from build123d import *

# Parameters (mm, degrees)
SKETCH1_R           = 7
BOSS_EXTRUDE1_DEPTH = 20
BOSS_EXTRUDE2_START = 1
SKETCH2_R           = 7
SKETCH2_R_2         = 2.05
BOSS_EXTRUDE2_DEPTH = 1


with BuildPart() as part:
    # Sketch1 → Boss-Extrude1 (new body)
    with BuildSketch(Plane(origin=(0, 0, 0), x_dir=(1, 0, 0), z_dir=(0, 1, 0))):
        with Locations(Location((0, 0, 0), (0, 0, 270))):
            Circle(SKETCH1_R)
        Polygon((0, 6.985938257), (-6.05, 3.492969129), (-6.05, -3.492969129), (0, -6.985938257), (6.05, -3.492969129), (6.05, 3.492969129), align=None, mode=Mode.SUBTRACT)
    extrude(amount=BOSS_EXTRUDE1_DEPTH)

    # Sketch2 → Boss-Extrude2 (add)
    with BuildSketch(Plane.XZ.offset(BOSS_EXTRUDE2_START)):
        with Locations(Location((0, 0, 0), (0, 0, 270))):
            Circle(SKETCH2_R)
        with Locations(Location((0, 0, 0), (0, 0, 270))):
            Circle(SKETCH2_R_2, mode=Mode.SUBTRACT)
    extrude(amount=-BOSS_EXTRUDE2_DEPTH)


solid = part.part
Geometry check sheet. Reference: the model listing, model coordinates, mm. A direction names the side the tool comes from. Round coordinates to 2 decimals unless told otherwise and drop trailing zeros. Order: outer loops, then holes, each group sorted by start corner. A loop starts at its lowest first (then second) coordinate and runs counter-clockwise, first axis right, second up. Notation, with made-up numbers: M 76.5,46.5 L 92.5,46.5 A20 ccw 92.5,68.5 Z; hole C 26.25,-22.75 d2. An arc over 180 degrees is marked long. Answer in a Markdown table with one row per item.
(1) Draft check along X on faces 3 (the face through (-3.067, 9.86, 5.215)), 4 (the face through (2, -1, -1)). Enter one of: released by +X, released by -X, zero draft, split by the parting line, or undercut.
Responses:
| item | result |
|---|---|
| face 3 | undercut |
| face 4 | zero draft |
(2) Sectioned sample at D-D, the plane x = -5. Record the cut outline in (y, z), and give its area (3 significant figures).
Responses:
| item | result |
|---|---|
| outline | M -1,-4.9 L 20,-4.9 L 20,-4.1 L 0,-4.1 L 0,4.1 L 20,4.1 L 20,4.9 L -1,4.9 Z |
| area | 41.8 mm² |
(3) Scan lines: probe 1 along X at (y, z) = (-0.65, 0); probe 2 along Y at (x, z) = (5, 0.75); probe 3 along Z at (x, y) = (3.5, 10). Record each from-to range of solid material in increasing order. Write a range as from..to.
Responses:
| item | result |
|---|---|
| probe 1 | x = -7..-2.05, 2.05..7 |
| probe 2 | y = -1..0 |
| probe 3 | z = -6.06..-4.97, 4.97..6.06 |
(4) Sectioned sample at C-C, the plane x = 1.5. Record the cut outline in (y, z), and give its area (3 significant figures).
Responses:
| item | result |
|---|---|
| outline | M -1,-6.84 L 20,-6.84 L 20,-6.12 L 0,-6.12 L 0,-1.4 L -1,-1.4 Z; M -1,1.4 L 0,1.4 L 0,6.12 L 20,6.12 L 20,6.84 L -1,6.84 Z |
| area | 39.6 mm² |
(5) Go/stop test with flat-tipped pins: P1, Ø8, axis at y = 16.5, z = 5, coming from the -X side; P2, Ø6, axis at x = 3, y = 17.5, coming from the -Z side; P3, Ø3, axis at y = 11, z = 3.5, coming from the -X side; P4, Ø6, axis at x = -4, y = 16, coming from the -Z side. Record where each tip stops, or that it passes through.
Responses:
| item | result |
|---|---|
| P1 | stops at x = -6.93 |
| P2 | stops at z = -7 |
| P3 | stops at x = -6.71 |
| P4 | stops at z = -6.93 |
(6) Sectioned sample at A-A, the plane z = 0. Record the cut outline in (x, y), and give its area (3 significant figures).
Responses:
| item | result |
|---|---|
| outline | M -7,-1 L -2.05,-1 L -2.05,0 L -6.05,0 L -6.05,20 L -7,20 Z; M 2.05,-1 L 7,-1 L 7,20 L 6.05,20 L 6.05,0 L 2.05,0 Z |
| area | 47.9 mm² |
(7) Tool access check on faces 1 (the face through (2.983, 9.86, 5.264)), 2 (the face through (2.033, -0.507, 0.267)). Record the directions out of +Z, -Z, +X, -X, +Y, -Y that give a thin tool (end or side, any length) a straight path to the whole face; none if there is none.
Responses:
| item | result |
|---|---|
| face 1 | +Y |
| face 2 | +Y, -Y |
(8) Sectioned sample at B-B, the plane y = 10. Record the cut outline in (x, z), and give its area (3 significant figures).
Responses:
| item | result |
|---|---|
| outline | C 0,0 d14; hole M -6.05,-3.49 L 0,-6.99 L 6.05,-3.49 L 6.05,3.49 L 0,6.99 L -6.05,3.49 Z |
| area | 27.1 mm² |
